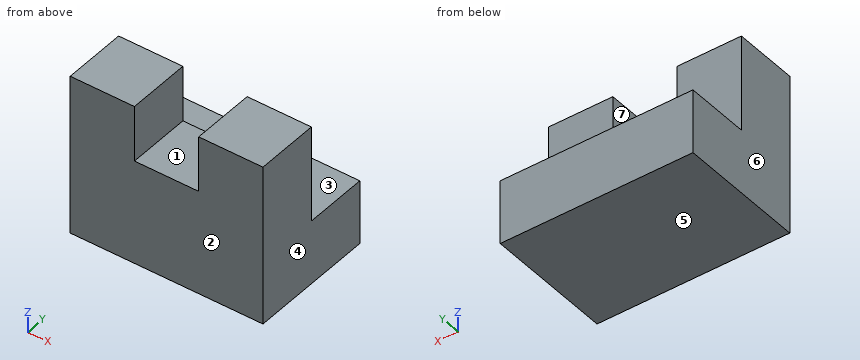
from build123d import *

# Parameters (mm, degrees)
F1_DEPTH = 25.4
F3_DEPTH = 12.7


with BuildPart() as f1:
    # F0 (on Front) → F1 (new body)
    with BuildSketch(Plane.XZ):
        Polygon((0, 31.75), (0, 0), (38.1, 0), (38.1, 31.75), (25.4, 31.75), (25.4, 20.713098), (12.7, 20.713098), (12.7, 31.75), align=None)
    extrude(amount=F1_DEPTH)

    # F2 (on face) → F3 (cut)
    with BuildSketch(Plane(origin=(0, 0, 0), x_dir=(-1, 0, 0), z_dir=(0, 1, 0))):
        Polygon((-38.1, 31.75), (-38.1, 12.7), (0, 12.7), (0, 31.75), (-12.7, 31.75), (-12.7, 20.713098), (-25.4, 20.713098), (-25.4, 31.75), align=None)
    extrude(amount=-F3_DEPTH, mode=Mode.SUBTRACT)


solid = f1.part
Design review of the part built by this model. Coordinates are the model's own, in mm. Face numbers are marked on the shaded views. A direction names the side the tool comes from. Give positions to 0.01 mm unless a question says otherwise; leave off trailing zeros. Write each loop counter-clockwise with the first axis right and the second up, starting at its lowest first coordinate (ties: lowest second). Pieces come first, ordered by that corner, then holes. Notation, with made-up numbers: M -33,23.5 L 22,23.5 A19 cw 22,46.5 Z; hole C 57.25,-2.75 d5. An arc over 180 degrees is marked long. Answer as a JSON object with one key per item and string values. Group by question number.
1) We need section A-A (z = 26.5). Give the boundary of the cut face in (x, y), and give its area (3 significant figures).
2) We need section C-C (x = 4). Give the boundary of the cut face in (y, z).
3) Mouldability with a two-part tool opening along X and no side actions: class the marked faces 4, 5, 6 and 7 as released by +X, released by -X, zero draft, split by the parting line, or undercut.
4) Tool access review of the marked faces 1, 2 and 3: name each direction out of +Z, -Z, +X, -X, +Y, -Y from which nothing blocks a thin tool from reaching the whole face with its end or side.
5) We need section D-D (z = 16.5). Give the boundary of the cut face in (x, y).
6) Clearance check with flat-ended pins moving along their axes: pin 1 Ø5.5 at (x, z) = (12.5, 18.5) entering from +Y; pin 2 Ø4 at (x, y) = (26, -4) entering from +Z. State where each tip first meets the part, or that it passes through.
7) We need section B-B (y = -15.5). Give the boundary of the cut face in (x, z), and give its area (3 significant figures).
8) For line 1 along X through (y, z) = (-14.75, 28.5); line 2 along Y through (x, z) = (5, 21.5); line 3 along Z through (x, y) = (16, -23.5), list the stretches that pass through material, from the lowest coordinate up.
Answer key:
{
 "1": {"outline": "M 0,-25.4 L 12.7,-25.4 L 12.7,-12.7 L 0,-12.7 Z; M 25.4,-25.4 L 38.1,-25.4 L 38.1,-12.7 L 25.4,-12.7 Z", "area": "323 mm²"},
 "2": {"outline": "M -25.4,0 L 0,0 L 0,12.7 L -12.7,12.7 L -12.7,31.75 L -25.4,31.75 Z"},
 "3": {"face 4": "released by +X", "face 5": "zero draft", "face 6": "released by -X", "face 7": "undercut"},
 "4": {"face 1": "+Z, +Y, -Y", "face 2": "+Z, -Z, +X, -X, -Y", "face 3": "+Z, +X, -X, +Y"},
 "5": {"outline": "M 0,-25.4 L 38.1,-25.4 L 38.1,-12.7 L 0,-12.7 Z"},
 "6": {"pin 1": "stops at y = -12.7", "pin 2": "stops at z = 12.7"},
 "7": {"outline": "M 0,0 L 38.1,0 L 38.1,31.75 L 25.4,31.75 L 25.4,20.71 L 12.7,20.71 L 12.7,31.75 L 0,31.75 Z", "area": "1,070 mm²"},
 "8": {"line 1": "x = 0 to 12.7, 25.4 to 38.1", "line 2": "y = -25.4 to -12.7", "line 3": "z = 0 to 20.71"}
}
